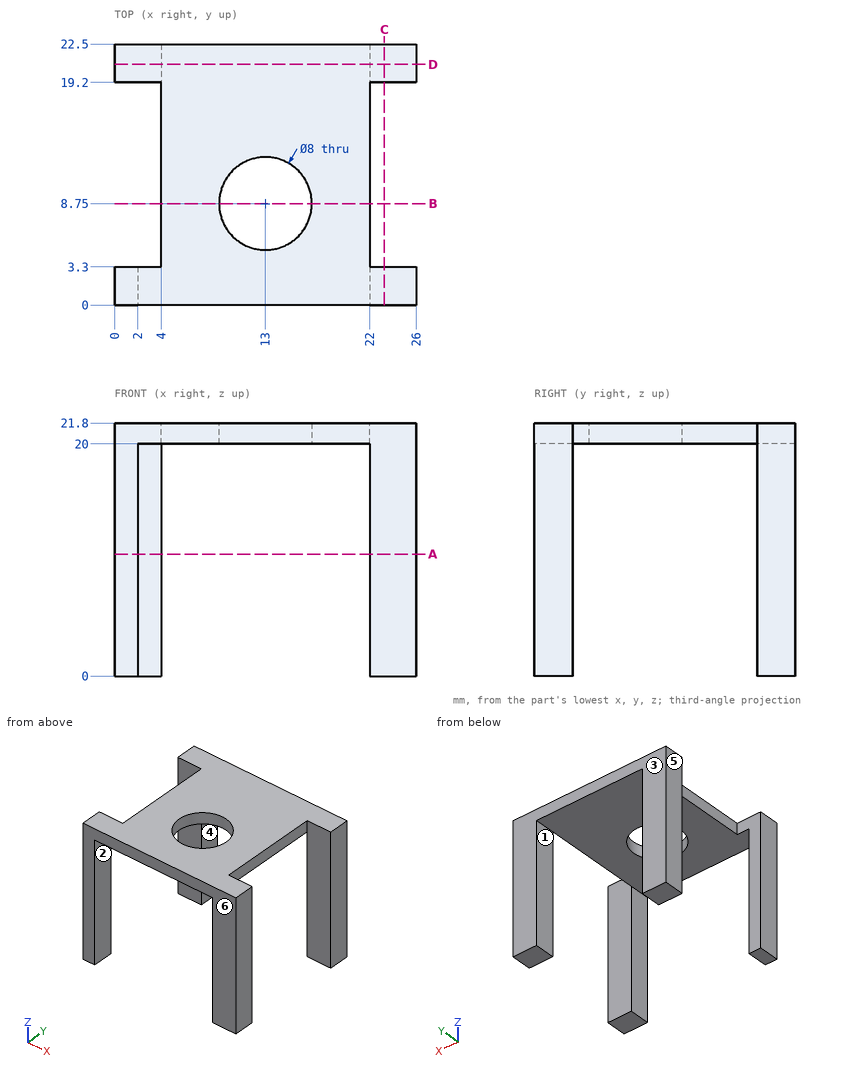
Answer from the drawing. Dimensions are ordinates in mm from the lowest x, y and z of the part. A direction names the side the tool comes from. Round coordinates to 2 decimals unless told otherwise and drop trailing zeros. Write each loop counter-clockwise with the first axis right and the second up, starting at its lowest first coordinate (ties: lowest second). Pieces come first, ordered by that corner, then holes. Notation, with made-up numbers: M 31,-38 L 56,-38 A16 cw 56,-23 Z; hole C 17.25,7 d10. An arc over 180 degrees is marked long. Write each question's results on one line, items separated by ' | '. Start each with the question number.
Item 1: Straight lines are drawn through the part: probe 1 along Y at (x, z) = (13, 20.55); probe 2 along Y at (x, z) = (23.5, 18); probe 3 along Z at (x, y) = (19.5, 16). For each, find the intervals that lie inside material, in ascending order.
Item 2: Given pin 1 Ø10 at (x, y) = (14.5, 16.5) entering from -Z; pin 2 Ø0.9 at (y, z) = (8, 20.5) entering from +X; pin 3 Ø0.9 at (y, z) = (12.5, 21) entering from -X, each flat-ended and moving along its own axis, determine where each tip first touches the part or whether it passes through.
Item 3: Find section A-A on z = 10.5. Write down the section's boundary in (x, y), and give its area (3 significant figures).
Item 4: Find section D-D on y = 20.75. Write down the section's boundary in (x, z).
Item 5: Find section C-C on x = 23.25. Write down the section's boundary in (y, z).
Item 6: Which of the six approach directions +Z, -Z, +X, -X, +Y, -Y give full straight-line access (tool end or side, diameter ignored) to the marked faces 1, 2 and 3?
Item 7: Find section B-B on y = 8.75. Write down the section's boundary in (x, z), and give its area (3 significant figures).
Item 8: The mould has two halves that part along X. Classify the marked faces 4, 5 and 6: +X half, -X half, draft (parallel to the pull), parting line (faces both ways), or undercut.
Answer block:
1) probe 1: y = 0 to 4.75, 12.75 to 22.5 | probe 2: y = 0 to 3.3, 19.2 to 22.5 | probe 3: z = 20 to 21.8
2) pin 1: stops at z = 20 | pin 2: stops at x = 22 | pin 3: stops at x = 4
3) outline: M 0,0 L 2,0 L 2,3.3 L 0,3.3 Z; M 0,19.2 L 4,19.2 L 4,22.5 L 0,22.5 Z; M 22,0 L 26,0 L 26,3.3 L 22,3.3 Z; M 22,19.2 L 26,19.2 L 26,22.5 L 22,22.5 Z | area: 46.2 mm²
4) outline: M 0,0 L 4,0 L 4,20 L 22,20 L 22,0 L 26,0 L 26,21.8 L 0,21.8 Z
5) outline: M 0,0 L 3.3,0 L 3.3,21.8 L 0,21.8 Z; M 19.2,0 L 22.5,0 L 22.5,21.8 L 19.2,21.8 Z
6) face 1: -Z, +Y, -Y | face 2: -Z, -Y | face 3: +Z, -Z, +X, -X, +Y
7) outline: M 4,20 L 9,20 L 9,21.8 L 4,21.8 Z; M 17,20 L 22,20 L 22,21.8 L 17,21.8 Z | area: 18.0 mm²
8) face 4: undercut | face 5: -X half | face 6: draft
